Design review of the part built by this model. Coordinates are the model's own, in mm. Face numbers are marked on the shaded views. A direction names the side the tool comes from. Round coordinates to 2 decimals unless told otherwise and drop trailing zeros. Loops run counter-clockwise (first coordinate to the right, second up) from the corner with the lowest first, then second, coordinate; pieces in that order, holes last. Notation, with made-up numbers: (51, -35.5) -> (80, -35.5) arc R10 cw to (80, -24.5) -> close; hole circle Ø4 at (-6.75, 60.25). An arc over 180 degrees is marked (long way). Write each question's results on one line, items separated by ' | '. Start each with the question number.
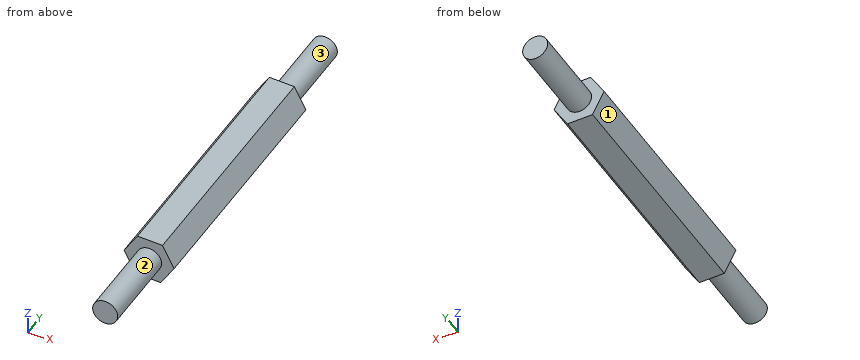
from build123d import *

# Parameters (mm, degrees)
BOSS_EXTRUDE1_DEPTH = 30
SKETCH4_R           = 1.5
BOSS_EXTRUDE2_DEPTH = 10
BOSS_EXTRUDE3_START = 10
SKETCH5_R           = 1.5
BOSS_EXTRUDE3_DEPTH = 10


with BuildPart() as part:
    # Sketch3 → Boss-Extrude1 (new body)
    with BuildSketch(Plane(origin=(0, 0, 0), x_dir=(1, 0, 0), z_dir=(0, 1, 0))):
        Polygon((1.388964752, 2.662182442), (-1.611035248, 2.533969981), (-3, -0.12821246), (-1.388964752, -2.662182442), (1.611035248, -2.533969981), (3, 0.12821246), align=None)
    extrude(amount=BOSS_EXTRUDE1_DEPTH)

    # Sketch4 → Boss-Extrude2 (add)
    with BuildSketch(Plane(origin=(0, 30, 0), x_dir=(1, 0, 0), z_dir=(0, 1, 0))):
        with Locations(Location((0, 0, 0), (0, 0, 270))):
            Circle(SKETCH4_R)
    extrude(amount=BOSS_EXTRUDE2_DEPTH)

    # Sketch5 → Boss-Extrude3 (add)
    with BuildSketch(Plane.XZ.offset(BOSS_EXTRUDE3_START)):
        with Locations(Location((0, 0, 0), (0, 0, 90))):
            Circle(SKETCH5_R)
    extrude(amount=-BOSS_EXTRUDE3_DEPTH)


solid = part.part
1) To check wall thickness, follow line 1 (Y direction, x = 1.35, z = -1.75); line 2 (Z direction, x = -0.1, y = -5.5); line 3 (X direction, y = 27.5, z = 2.05). State the ranges of each line that lie inside material, in increasing order. Write a range as from..to.
2) For the marked faces 1, 2 and 3, list the 3-axis set-ups (+Z, -Z, +X, -X, +Y, -Y) from which the entire face can be reached by the end or side of a thin tool; tool diameter is ignored.
3) Take a section at C-C (y = -3). Write out the cut boundary in (x, z).
4) Take a section at A-A (z = -1.05). Write out the cut boundary in (x, y).
5) Take a section at D-D (z = 1.95). Write out the cut boundary in (x, y).
6) Take a section at B-B (x = 0). Write out the cut boundary in (y, z), plus the area to 3 significant figures.
7) Insertion check: pin 1 (1.5 mm diameter, centred on x = -2, y = 0, fed in from +Z). The pin has a flat end and moves straight along its axis. Give the tip position at first contact, or say it passes through.
Geometry check:
1) line 1: y = 0..30 | line 2: z = -1.5..1.5 | line 3: x = -1.78..1.86
2) face 1: -Z, -X, +Y, -Y | face 2: -Y | face 3: +Y
3) outline: circle Ø3 at (0, 0)
4) outline: (-2.39, 0) -> (-1.07, 0) -> (-1.07, -10) -> (1.07, -10) -> (1.07, 0) -> (2.41, 0) -> (2.41, 30) -> (1.07, 30) -> (1.07, 40) -> (-1.07, 40) -> (-1.07, 30) -> (-2.39, 30) -> close
5) outline: (-1.84, 0) -> (1.92, 0) -> (1.92, 30) -> (-1.84, 30) -> close
6) outline: (-10, -1.5) -> (0, -1.5) -> (0, -2.6) -> (30, -2.6) -> (30, -1.5) -> (40, -1.5) -> (40, 1.5) -> (30, 1.5) -> (30, 2.6) -> (0, 2.6) -> (0, 1.5) -> (-10, 1.5) -> close | area: 216 mm^2
7) pin 1: stops at z = 2.66
